from build123d import *

# Parameters (mm, degrees)
F0_R     = 2
F1_DEPTH = 86
F2_R     = 19
F3_DEPTH = 2
F4_R     = 3.175
F5_DEPTH = 21
F6_R     = 0.5
F8_R     = 9
F9_DEPTH = 83
F10_R    = 3


# Not quite as in the source:
# - a feature names something its author has since deleted; it is built from what else it names


with BuildPart() as f1:
    # F0 (on Right) → F1 (new body)
    with BuildSketch(Plane.YZ):
        with BuildLine():
            Line((26.1, 28.1), (-26.1, 28.1))
            ThreePointArc((-26.1, 28.1), (-27.5142135624, 27.5142135624), (-28.1, 26.1))
            Line((-28.1, 26.1), (-28.1, -26.1))
            ThreePointArc((-28.1, -26.1), (-27.5142135624, -27.5142135624), (-26.1, -28.1))
            Line((-26.1, -28.1), (26.1, -28.1))
            ThreePointArc((26.1, -28.1), (27.5142135624, -27.5142135624), (28.1, -26.1))
            Line((28.1, -26.1), (28.1, 26.1))
            ThreePointArc((28.1, 26.1), (27.5142135624, 27.5142135624), (26.1, 28.1))
        make_face()
        with Locations((-23.5, -23.5)):
            Circle(F0_R, mode=Mode.SUBTRACT)
        with Locations((23.5, -23.5)):
            Circle(F0_R, mode=Mode.SUBTRACT)
        with Locations((-23.5, 23.5)):
            Circle(F0_R, mode=Mode.SUBTRACT)
        with Locations((23.5, 23.5)):
            Circle(F0_R, mode=Mode.SUBTRACT)
    extrude(amount=F1_DEPTH)

    # F2 (on face) → F3 (join)
    with BuildSketch(Plane.YZ.offset(86)):
        Circle(F2_R)
    extrude(amount=F3_DEPTH)

    # F4 (on face) → F5 (join)
    with BuildSketch(Plane.YZ.offset(88)):
        Circle(F4_R)
    extrude(amount=F5_DEPTH)

    # F6
    f6_edges = [f1.edges().sort_by_distance(p)[0] for p in [
        (109, -3.175, 0),
    ]]
    fillet(f6_edges, radius=F6_R)

    # F8 (on offset) → F9 (cut, through all)
    with BuildSketch(Plane.YZ.offset(83)):
        with Locations((-26.1, 26.1)):
            Circle(F8_R)
        with Locations((26.1, 26.1)):
            Circle(F8_R)
        with Locations((-26.1, -26.1)):
            Circle(F8_R)
        with Locations((26.1, -26.1)):
            Circle(F8_R)
    extrude(amount=-F9_DEPTH, mode=Mode.SUBTRACT)

    # F10
    f10_edges = [f1.edges().sort_by_distance(p)[0] for p in [
        (41.5, 17.325036, 28.1),
        (41.5, 28.1, 17.325036),
        (41.5, -17.325036, 28.1),
        (41.5, -28.1, 17.325036),
        (41.5, -28.1, -17.325036),
        (41.5, -17.325036, -28.1),
        (41.5, 17.325036, -28.1),
        (41.5, 28.1, -17.325036),
    ]]
    fillet(f10_edges, radius=F10_R)


solid = f1.part
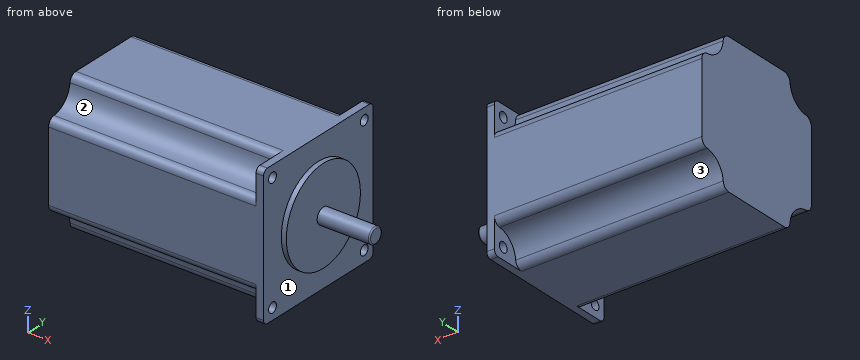
Build history of the part. All positions in model axes, mm. Face numbers are marked on the shaded views. A direction names the side the tool comes from. Round coordinates to 2 decimals unless told otherwise and drop trailing zeros. Write each loop counter-clockwise with the first axis right and the second up, starting at its lowest first coordinate (ties: lowest second). Pieces come first, ordered by that corner, then holes. Notation, with made-up numbers: M 45.5,4 L 64.5,4 A4 ccw 64.5,9 Z; hole C -28,21 d1. An arc over 180 degrees is marked long. Answer as a JSON object with one key per item and string values. Group by question number.
(1) Cut at C-C (z = 0). Give the cut face in (x, y) (3 decimals), and give its area (3 significant figures).
(2) Drill centre lines: L1, parallel to Z at x = 84.2, y = 23.5; L2, parallel to Z at x = 84, y = 23. Where is each one in solid material? Low to high.
(3) Cut at A-A (y = 23.5). Give the cut face in (x, z).
(4) Flat gauge pins, fed straight in: pin 1 (5 mm diameter, centred on y = -23.5, z = -23.5, fed in from -X); pin 2 (10 mm diameter, centred on y = 5, z = -9, fed in from +X); pin 3 (1 mm diameter, centred on x = 17, y = -21, fed in from +Z). Where does each tip first touch, or does it go through?
(5) Cut at B-B (x = 56). Give the cut face in (y, z), and give its area (3 significant figures).
(6) Which spindle directions (+Z, -Z, +X, -X, +Y, -Y) get a long thin tool onto all of the face, cutting with end or side? Do the marked faces 1, 2 and 3. Say none if no direction does.
Responses:
{
 "1": {"outline": "M 0,-28.1 L 86,-28.1 L 86,-19 L 88,-19 L 88,-3.175 L 108.5,-3.175 A0.5 ccw 109,-2.675 L 109,2.675 A0.5 ccw 108.5,3.175 L 88,3.175 L 88,19 L 86,19 L 86,28.1 L 0,28.1 Z", "area": "5,040 mm2"},
 "2": {"L1": "z = -28.1 to -25.5, -21.5 to 21.5, 25.5 to 28.1", "L2": "z = -28.1 to -25.44, -21.56 to 21.56, 25.44 to 28.1"},
 "3": {"outline": "M 0,-17.48 L 83,-17.48 L 83,-21.5 L 86,-21.5 L 86,21.5 L 83,21.5 L 83,17.48 L 0,17.48 Z; M 83,-28.1 L 86,-28.1 L 86,-25.5 L 83,-25.5 Z; M 83,25.5 L 86,25.5 L 86,28.1 L 83,28.1 Z"},
 "4": {"pin 1": "stops at x = 83", "pin 2": "stops at x = 88", "pin 3": "stops at z = 19.05"},
 "5": {"outline": "M -28.1,-14.14 A3 ccw -25.35,-17.13 A9 cw -17.13,-25.35 A3 ccw -14.14,-28.1 L 14.14,-28.1 A3 ccw 17.13,-25.35 A9 cw 25.35,-17.13 A3 ccw 28.1,-14.14 L 28.1,14.14 A3 ccw 25.35,17.13 A9 cw 17.13,25.35 A3 ccw 14.14,28.1 L -14.14,28.1 A3 ccw -17.13,25.35 A9 cw -25.35,17.13 A3 ccw -28.1,14.14 Z", "area": "2,730 mm2"},
 "6": {"face 1": "+X", "face 2": "+Z, -X, -Y", "face 3": "-Z, -X, +Y"}
}
